The listing builds one solid part. Answer for the finished solid, in the listing's coordinates (mm). A direction names the side the tool comes from. Coordinates: 2 decimals unless noted, no trailing zeros. Write each loop counter-clockwise with the first axis right and the second up, starting at its lowest first coordinate (ties: lowest second). Pieces come first, ordered by that corner, then holes. Notation, with made-up numbers: M 49,30 L 86,30 A11 cw 86,43 Z; hole C 85,67.5 d9. An arc over 180 degrees is marked long. Answer as a JSON object with one key per item and string values. Group by question number.
from build123d import *

# Parameters (mm, degrees)
BOSS_EXTRUDE1_DEPTH = 16
SKETCH2_R           = 4
CUT_EXTRUDE1_DEPTH  = 87.492774265
SKETCH3_R           = 5
CUT_EXTRUDE2_DEPTH  = 32


with BuildPart() as part:
    # Sketch1 → Boss-Extrude1 (new, symmetric)
    with BuildSketch(Plane.XY):
        Polygon((-22.5, 0), (-22.5, 65), (22.5, 65), (22.5, 0), (25.5, 0), (25.5, 68), (-25.5, 68), (-25.5, 0), align=None)
    extrude(amount=BOSS_EXTRUDE1_DEPTH, both=True)

    # Sketch2 → Cut-Extrude1 (cut, through all)
    with BuildSketch(Plane(origin=(25.5, 0, 0), x_dir=(0, 0, -1), z_dir=(1, 0, 0))):
        with Locations((0, 10)):
            Circle(SKETCH2_R)
    extrude(amount=-CUT_EXTRUDE1_DEPTH, mode=Mode.SUBTRACT)

    # Sketch3 → Cut-Extrude2 (cut)
    with BuildSketch(Plane(origin=(0, 68, 0), x_dir=(1, 0, 0), z_dir=(0, 1, 0))):
        with Locations(Location((0, 0, 0), (0, 0, 270))):
            Circle(SKETCH3_R)
    extrude(amount=-CUT_EXTRUDE2_DEPTH, mode=Mode.SUBTRACT)


solid = part.part
Item 1: For a pull along Y with two mould halves and no side action, classify faces 3 (the face through (-5.3, 65, 0.2)), 4 (the face through (-4.88, 66.52, -1.08)), 5 (the face through (-23.979, 13.966, 0.521)), 6 (the face through (24.021, 13.966, 0.521)) as +Y half, -Y half, draft (parallel to the pull), parting line (faces both ways), or undercut.
Item 2: A tool of negligible diameter and unlimited length cuts with its end or side. For faces 1 (the face through (22.5, 33, 0)), 2 (the face through (-23, 39, 16)), from which of +Z, -Z, +X, -X, +Y, -Y can it reach the whole face along a straight path? Write none if from no direction.
Item 3: A cutting plane is placed at B-B, the plane x = 0. Write down the section's boundary in (y, z).
Item 4: Consider L1, parallel to X at y = 28, z = -8; L2, parallel to X at y = 66.85, z = 0; L3, parallel to Y at x = 24.4, z = 0. Determine where each line is inside the solid, lowest interval first. Write a range as from..to.
Item 5: A cutting plane is placed at A-A, the plane z = 0. Write down the section's boundary in (x, y).
Item 6: A cutting plane is placed at C-C, the plane y = 10. Write down the section's boundary in (x, z), and give its area (3 significant figures).
Item 7: A flat-ended cylindrical pin translates along its axis: pin 1 Ø1.5 at (x, z) = (-12.5, 10) entering from -Y. Find the tip coordinate at first contact, or state that the pin passes through.
Item 8: A cutting plane is placed at D-D, the plane y = 25.5. Write down the section's boundary in (x, z), and give its area (3 significant figures).
Answer:
{
 "1": {"face 3": "-Y half", "face 4": "draft", "face 5": "undercut", "face 6": "undercut"},
 "2": {"face 1": "+Z, -Z, -Y", "face 2": "+Z, +X, -X, +Y, -Y"},
 "3": {"outline": "M 65,-16 L 68,-16 L 68,-5 L 65,-5 Z; M 65,5 L 68,5 L 68,16 L 65,16 Z"},
 "4": {"L1": "-25.5..-22.5, 22.5..25.5", "L2": "-25.5..-5, 5..25.5", "L3": "0..6, 14..68"},
 "5": {"outline": "M -25.5,0 L -22.5,0 L -22.5,6 L -25.5,6 Z; M -25.5,14 L -22.5,14 L -22.5,65 L -5,65 L -5,68 L -25.5,68 Z; M 5,65 L 22.5,65 L 22.5,14 L 25.5,14 L 25.5,68 L 5,68 Z; M 22.5,0 L 25.5,0 L 25.5,6 L 22.5,6 Z"},
 "6": {"outline": "M -25.5,-16 L -22.5,-16 L -22.5,-4 L -25.5,-4 Z; M -25.5,4 L -22.5,4 L -22.5,16 L -25.5,16 Z; M 22.5,-16 L 25.5,-16 L 25.5,-4 L 22.5,-4 Z; M 22.5,4 L 25.5,4 L 25.5,16 L 22.5,16 Z", "area": "144 mm2"},
 "7": {"pin 1": "y = 65"},
 "8": {"outline": "M -25.5,-16 L -22.5,-16 L -22.5,16 L -25.5,16 Z; M 22.5,-16 L 25.5,-16 L 25.5,16 L 22.5,16 Z", "area": "192 mm2"}
}
